The model under review builds one solid part; all positions refer to its coordinate system, in mm. Face numbers are marked on the shaded views. A direction names the side the tool comes from. Give positions to 0.01 mm unless a question says otherwise; leave off trailing zeros. Order: outer loops, then holes, each group sorted by start corner. A loop starts at its lowest first (then second) coordinate and runs counter-clockwise, first axis right, second up.
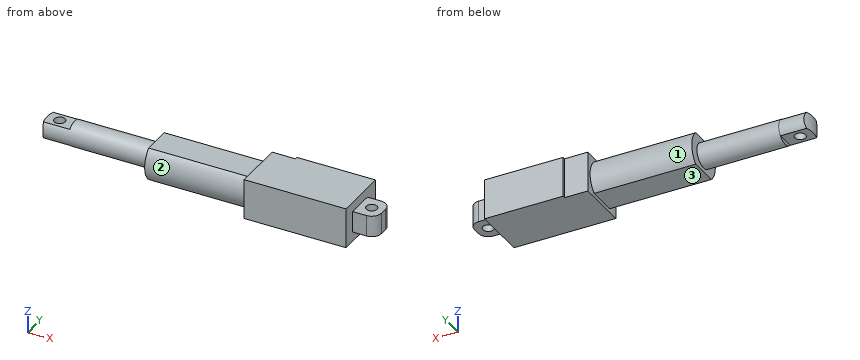
```python
from build123d import *

# Parameters (mm, degrees)
PAD001_DEPTH = 14.8
SKETCH004_R  = 2
PAD002_DEPTH = 7.8
PAD003_DEPTH = 37.3
SKETCH008_R  = 4.5
PAD004_DEPTH = 30
PAD005_DEPTH = 11
SKETCH007_R  = 2
POCKET_DEPTH = 14.801


with BuildPart() as part:
    # Sketch003 → Pad001 (new body)
    with BuildSketch(Plane.XY):
        Polygon((0, 0), (37.4, 0), (37.4, 20), (8.5, 20), (8.5, 19), (0, 19), align=None)
    extrude(amount=PAD001_DEPTH)

    # Sketch004 → Pad002 (join)
    with BuildSketch(Plane.XY.offset(3.5)):
        with BuildLine():
            Line((37.4, 14.5), (42.5, 14.5))
            ThreePointArc((46, 11), (44.9748737342, 13.4748737342), (42.5, 14.5))
            Line((46, 11), (46, 8))
            ThreePointArc((42.5, 4.5), (44.9748737342, 5.5251262658), (46, 8))
            Line((42.5, 4.5), (37.4, 4.5))
            Line((37.4, 4.5), (37.4, 14.5))
        make_face()
        with Locations((41.7, 9.5)):
            Circle(SKETCH004_R, mode=Mode.SUBTRACT)
    extrude(amount=PAD002_DEPTH)

    # Sketch005 → Pad003 (join)
    with BuildSketch(Plane(origin=(0, 0, 0), x_dir=(0, -1, 0), z_dir=(-1, 0, 0))):
        with BuildLine():
            Line((-4.2084973779, 13.4), (-14.7915026221, 13.4))
            ThreePointArc((-14.7915026221, 13.4), (-17.5, 7.4), (-14.7915026221, 1.4))
            Line((-14.7915026221, 1.4), (-4.2084973779, 1.4))
            ThreePointArc((-4.2084973779, 1.4), (-1.5, 7.4), (-4.2084973779, 13.4))
        make_face()
    extrude(amount=PAD003_DEPTH)

    # Sketch008 (on Face17 of Pad003) → Pad004 (join)
    with BuildSketch(Plane(origin=(-37.3, 0, 0), x_dir=(0, -1, 0), z_dir=(-1, 0, 0))):
        with Locations((-9.5, 7.4)):
            Circle(SKETCH008_R)
    extrude(amount=PAD004_DEPTH)

    # Sketch006 (on Face17 of Pad003) → Pad005 (join)
    with BuildSketch(Plane(origin=(-67.3, 0, 0), x_dir=(0, -1, 0), z_dir=(-1, 0, 0))):
        with BuildLine():
            Line((-6.1912993487, 10.45), (-12.8087006513, 10.45))
            ThreePointArc((-12.8087006513, 10.45), (-14, 7.4), (-12.8087006513, 4.35))
            Line((-12.8087006513, 4.35), (-6.1912993487, 4.35))
            ThreePointArc((-6.1912993487, 4.35), (-5, 7.4), (-6.1912993487, 10.45))
        make_face()
    extrude(amount=PAD005_DEPTH)

    # Sketch007 → Pocket (cut, through all)
    with BuildSketch(Plane.XY):
        with Locations((-72.8, 9.5)):
            Circle(SKETCH007_R)
        with BuildLine():
            ThreePointArc((-76.5, 14), (-77.5, 9.5), (-76.5, 5))
            Line((-86.5, 5), (-76.5, 5))
            Line((-86.5, 14), (-86.5, 5))
            Line((-76.5, 14), (-86.5, 14))
        make_face()
    extrude(amount=POCKET_DEPTH, mode=Mode.SUBTRACT)


with BuildPart() as part_1:
    # Body002 placement: moved
    add(part.part.moved(Location((-41.7, -9.5, 0))))


solid = part_1.part
```
1. For the marked faces 1, 2 and 3, list the 3-axis set-ups (+Z, -Z, +X, -X, +Y, -Y) from which the entire face can be reached by the end or side of a thin tool; tool diameter is ignored.
2. To check wall thickness, follow line 1 (Y direction, x = 0, z = 9.5); line 2 (Y direction, x = -36.5, z = 1); line 3 (Z direction, x = -63.5, y = 2). State the ranges of each line that lie inside material, in increasing order.
3. Take a section at D-D (x = -51.5). Write out the cut boundary in (y, z), and give its area (3 significant figures).
4. Take a section at B-B (x = -114.5). Write out the cut boundary in (y, z), and give its area (3 significant figures).
5. Take a section at A-A (y = 0). Write out the cut boundary in (x, z), and give its area (3 significant figures).
6. Insertion check: pin 1 (1 mm diameter, centred on y = 2, z = 9, fed in from -X); pin 2 (2 mm diameter, centred on x = -47.5, z = 13, fed in from +Y); pin 3 (8.5 mm diameter, centred on x = -63.5, y = 0, fed in from -Z). Each pin has a flat end and moves straight along its axis. Give the tip position at first contact, or say it passes through.
7. Take a section at C-C (z = 7.4). Write out the cut boundary in (x, y) (3 decimals), and give its area (3 significant figures).
Answer:
1. face 1: -X, +Y
1. face 2: -X, -Y
1. face 3: -Z, -X, +Y, -Y
2. line 1: y = -5 to -2, 2 to 5
2. line 2: y = -9.5 to 9.5
2. line 3: z = 1.4 to 13.4
3. outline: (-5.29, 1.4) - (5.29, 1.4) arc R8 ccw to (5.29, 13.4) - (-5.29, 13.4) arc R8 ccw to start
3. area: 172 mm2
4. outline: (-3.31, 4.35) - (-2, 4.35) - (-2, 10.45) - (-3.31, 10.45) arc R4.5 ccw to start; (2, 4.35) - (3.31, 4.35) arc R4.5 ccw to (3.31, 10.45) - (2, 10.45) - close
4. area: 25.9 mm2
5. outline: (-119.2, 4.35) - (-116.5, 4.35) - (-116.5, 10.45) - (-119.2, 10.45) - close; (-112.5, 4.35) - (-109, 4.35) - (-109, 2.9) - (-79, 2.9) - (-79, 1.4) - (-41.7, 1.4) - (-41.7, 0) - (-4.3, 0) - (-4.3, 3.5) - (-2, 3.5) - (-2, 11.3) - (-4.3, 11.3) - (-4.3, 14.8) - (-41.7, 14.8) - (-41.7, 13.4) - (-79, 13.4) - (-79, 11.9) - (-109, 11.9) - (-109, 10.45) - (-112.5, 10.45) - close; (2, 3.5) - (4.3, 3.5) - (4.3, 11.3) - (2, 11.3) - close
5. area: 1,340 mm2
6. pin 1: stops at x = -119.09
6. pin 2: stops at y = 6.55
6. pin 3: stops at z = 1.4
7. outline: (-118.2, -4.5) - (-79, -4.5) - (-79, -8) - (-41.7, -8) - (-41.7, -9.5) - (-4.3, -9.5) - (-4.3, -5) - (0.8, -5) arc R3.5 ccw to (4.3, -1.5) - (4.3, 1.5) arc R3.5 ccw to (0.8, 5) - (-4.3, 5) - (-4.3, 10.5) - (-33.2, 10.5) - (-33.2, 9.5) - (-41.7, 9.5) - (-41.7, 8) - (-79, 8) - (-79, 4.5) - (-118.2, 4.5) arc R10.625 ccw to start; hole circle Ø4 at (-114.5, 0); hole circle Ø4 at (0, 0)
7. area: 1,750 mm2
